```python
from build123d import *

# Parameters (mm, degrees)
SKETCH1_W           = 20
SKETCH1_H           = 45.1
SKETCH1_R           = 1
SKETCH1_R_2         = 0.65
BOSS_EXTRUDE1_DEPTH = 1.6
SKETCH2_W           = 15.7
SKETCH2_H           = 6
BOSS_EXTRUDE2_DEPTH = 8.6
CUT_EXTRUDE1_DEPTH  = 18.3
SKETCH4_W           = 2.2
SKETCH4_H           = 3.601430215
CUT_EXTRUDE2_DEPTH  = 4
SKETCH5_R           = 0.95
CUT_EXTRUDE3_DEPTH  = 0.1
SKETCH6_W           = 2.7
SKETCH6_H           = 4.21
BOSS_EXTRUDE3_DEPTH = 1.5
SKETCH7_RX          = 1.124329337
SKETCH7_RY          = 0.743812381
BOSS_EXTRUDE4_DEPTH = 0.6
BOSS_EXTRUDE5_DEPTH = 3
BOSS_EXTRUDE6_DEPTH = 12.8
SKETCH10_W          = 9
SKETCH10_H          = 8
BOSS_EXTRUDE7_DEPTH = 3.65


with BuildPart() as part:
    # Sketch1 → Boss-Extrude1 (new body)
    with BuildSketch(Plane(origin=(0, 0, 0), x_dir=(1, 0, 0), z_dir=(0, 1, 0))):
        with Locations((10, 22.55)):
            Rectangle(SKETCH1_W, SKETCH1_H)
        with Locations(Location((2.2, 43.4, 0), (0, 0, 270))):  # turned: the seam where the file's is
            Circle(SKETCH1_R, mode=Mode.SUBTRACT)
        with Locations(Location((17.65, 10.75, 0), (0, 0, 270))):  # turned: the seam where the file's is
            Circle(SKETCH1_R, mode=Mode.SUBTRACT)
        with Locations(Location((18, 4.55, 0), (0, 0, 270))):  # turned: the seam where the file's is
            Circle(SKETCH1_R_2, mode=Mode.SUBTRACT)
    extrude(amount=BOSS_EXTRUDE1_DEPTH)

    # Sketch2 → Boss-Extrude2 (add)
    with BuildSketch(Plane(origin=(0, 1.6, 0), x_dir=(1, 0, 0), z_dir=(0, 1, 0))):
        with Locations((9.45, 4.7)):
            Rectangle(SKETCH2_W, SKETCH2_H)
    extrude(amount=BOSS_EXTRUDE2_DEPTH)

    # Sketch3 → Cut-Extrude1 (cut, through all)
    with BuildSketch(Plane(origin=(17.3, 0, 0), x_dir=(0, 0, -1), z_dir=(1, 0, 0))):
        Polygon((1.7, 6.6), (2.2, 6.6), (3.3, 10.2), (1.7, 10.2), align=None)
        Polygon((6.063741388, 10.2), (7.7, 10.2), (7.7, 4.901672733), align=None)
    extrude(amount=-CUT_EXTRUDE1_DEPTH, mode=Mode.SUBTRACT)

    # Sketch4 → Cut-Extrude2 (cut)
    with BuildSketch(Plane.XY.offset(-1.7)):
        with Locations((5.735754943, 4.083777336)):
            Rectangle(SKETCH4_W, SKETCH4_H)
        with Locations((3.235754943, 4.083777336)):
            Rectangle(SKETCH4_W, SKETCH4_H)
        with Locations((8.235754943, 4.083777336)):
            Rectangle(SKETCH4_W, SKETCH4_H)
        with Locations((10.735754943, 4.083777336)):
            Rectangle(SKETCH4_W, SKETCH4_H)
        with Locations((13.235754943, 4.083777336)):
            Rectangle(SKETCH4_W, SKETCH4_H)
        with Locations((15.735754943, 4.083777336)):
            Rectangle(SKETCH4_W, SKETCH4_H)
    extrude(amount=-CUT_EXTRUDE2_DEPTH, mode=Mode.SUBTRACT)

    # Sketch5 → Cut-Extrude3 (cut)
    with BuildSketch(Plane(origin=(0, 10.2, 0), x_dir=(1, 0, 0), z_dir=(0, 1, 0))):
        with Locations(Location((3.235754943, 4.681870694, 0), (0, 0, 270))):  # turned: the seam where the file's is
            Circle(SKETCH5_R)
        with Locations(Location((5.735754943, 4.681870694, 0), (0, 0, 270))):  # turned: the seam where the file's is
            Circle(SKETCH5_R)
        with Locations(Location((8.235754943, 4.681870694, 0), (0, 0, 270))):  # turned: the seam where the file's is
            Circle(SKETCH5_R)
        with Locations(Location((10.735754943, 4.681870694, 0), (0, 0, 270))):  # turned: the seam where the file's is
            Circle(SKETCH5_R)
        with Locations(Location((13.235754943, 4.681870694, 0), (0, 0, 270))):  # turned: the seam where the file's is
            Circle(SKETCH5_R)
        with Locations(Location((15.735754943, 4.681870694, 0), (0, 0, 270))):  # turned: the seam where the file's is
            Circle(SKETCH5_R)
    extrude(amount=-CUT_EXTRUDE3_DEPTH, mode=Mode.SUBTRACT)

    # Sketch6 → Boss-Extrude3 (add)
    with BuildSketch(Plane(origin=(0, 1.6, 0), x_dir=(1, 0, 0), z_dir=(0, 1, 0))):
        with Locations((2.35, 15.605)):
            Rectangle(SKETCH6_W, SKETCH6_H)
    extrude(amount=BOSS_EXTRUDE3_DEPTH)

    # Sketch7 → Boss-Extrude4 (add)
    with BuildSketch(Plane(origin=(0, 3.1, 0), x_dir=(1, 0, 0), z_dir=(0, 1, 0))):
        with Locations(Location((2.35, 15.605), (0, 0, 90))):
            Ellipse(SKETCH7_RX, SKETCH7_RY)
    extrude(amount=BOSS_EXTRUDE4_DEPTH)

    # Sketch8 → Boss-Extrude5 (add)
    with BuildSketch(Plane(origin=(0, 1.6, 0), x_dir=(1, 0, 0), z_dir=(0, 1, 0))):
        with BuildLine():
            Line((17.281101187, 13.5), (19.8, 13.5))
            Line((19.8, 13.5), (19.8, 18.5))
            Line((19.8, 18.5), (17.281101187, 18.5))
            ThreePointArc((17.281101187, 18.5), (9.875, 16), (17.281101187, 13.5))
        make_face()
    extrude(amount=BOSS_EXTRUDE5_DEPTH)

    # Sketch9 → Boss-Extrude6 (add)
    with BuildSketch(Plane(origin=(15.5, 0, 0), x_dir=(0, 0, -1), z_dir=(1, 0, 0))):
        with BuildLine():
            Line((22.825, 6.8), (28.125, 6.8))
            ThreePointArc((28.125, 6.8), (30.725, 4.2), (28.125, 1.6))
            Line((28.125, 1.6), (22.825, 1.6))
            ThreePointArc((22.825, 1.6), (20.225, 4.2), (22.825, 6.8))
        make_face()
    extrude(amount=-BOSS_EXTRUDE6_DEPTH)

    # Sketch10 → Boss-Extrude7 (add)
    with BuildSketch(Plane(origin=(0, 1.6, 0), x_dir=(1, 0, 0), z_dir=(0, 1, 0))):
        with Locations((4.51, 35.55)):
            Rectangle(SKETCH10_W, SKETCH10_H)
    extrude(amount=BOSS_EXTRUDE7_DEPTH)


solid = part.part
```
The listing builds one solid part. Answer for the finished solid, in the listing's coordinates (mm). A direction names the side the tool comes from. Give positions to 0.01 mm unless a question says otherwise; leave off trailing zeros. Order: outer loops, then holes, each group sorted by start corner. A loop starts at its lowest first (then second) coordinate and runs counter-clockwise, first axis right, second up. Notation, with made-up numbers: (-26, 48) -> (29, 48) arc R10 cw to (29, 55) -> close; hole circle Ø8 at (12.25, -16.5). An arc over 180 degrees is marked (long way). Answer as a JSON object with one key per item and string values. Group by question number.
Item 1: A tool of negligible diameter and unlimited length cuts with its end or side. For faces 4 (the flat face through (4.336, 4, -4)), 5 (the flat face through (13, 10.1, -5)), 6 (the flat face through (1, 2, -16)), 7 (the flat face through (15, 4.6, -16)), from which of +Z, -Z, +X, -X, +Y, -Y can it reach the whole face along a straight path? Write none if from no direction.
Item 2: The part is cut by section A-A on z = -10.75. Write down the section's boundary in (x, y).
Item 3: The part is cut by section C-C on z = -4.55. Give the number of separate pieces and of enclosed holes in the cut face, and give its area (3 significant figures).
Item 4: The part is cut by section B-B on z = -24.5. Write down the section's boundary in (x, y).
Item 5: Determine the mould class of faces 1 (the flat face through (11.836, 4, -4)), 2 (the flat face through (8, 10.1, -5)), 3 (the flat face through (9.01, 3, -35)) for opening direction Y: pulls with the +Y half, pulls with the -Y half, needs draft (parallel to the pull), parting line crosses it, or undercut.
Item 6: Consider L1, parallel to Y at x = 3.25, z = -12; L2, parallel to Y at x = 13.25, z = -12; L3, parallel to X at y = 0.45, z = -43.4. Determine where each line is inside the solid, lowest interval first. Write a range as from..to.
Item 7: Flat-ended cylindrical pins translate along their axes: pin 1 (4 mm diameter, centred on x = 3, y = 8, fed in from +Z); pin 2 (0.7 mm diameter, centred on x = 3.5, z = -4.5, fed in from +Y); pin 3 (4 mm diameter, centred on y = 4, z = -3.5, fed in from -X). Find the tip coordinate at first contact, or state that the pin passes through.
Result set:
{
 "1": {"face 4": "+Z", "face 5": "+Y", "face 6": "+Z, -X, +Y", "face 7": "+X, -X, +Y"},
 "2": {"outline": "(0, 0) -> (16.65, 0) -> (16.65, 1.6) -> (0, 1.6) -> close; (18.65, 0) -> (20, 0) -> (20, 1.6) -> (18.65, 1.6) -> close"},
 "3": {"separate pieces": "2", "enclosed holes": "6", "area": "116 mm²"},
 "4": {"outline": "(0, 0) -> (20, 0) -> (20, 1.6) -> (15.5, 1.6) -> (15.5, 6.8) -> (2.7, 6.8) -> (2.7, 1.6) -> (0, 1.6) -> close"},
 "5": {"face 1": "undercut", "face 2": "pulls with the +Y half", "face 3": "needs draft"},
 "6": {"L1": "0..1.6", "L2": "0..4.6", "L3": "0..1.2, 3.2..20"},
 "7": {"pin 1": "z = -1.7", "pin 2": "y = 10.1", "pin 3": "x = 1.6"}
}
